```python
from build123d import *

# Parameters (mm, degrees)
BOSS_EXTRUDE1_DEPTH = 30
CUT_EXTRUDE1_DEPTH  = 59
SKETCH4_W           = 36.590571665
SKETCH4_H           = 16.65
BOSS_EXTRUDE2_DEPTH = 9
SKETCH5_W           = 22.6
SKETCH5_H           = 11.85
CUT_EXTRUDE2_DEPTH  = 4.3
CUT_EXTRUDE3_DEPTH  = 10.2
BOSS_EXTRUDE3_DEPTH = 27
SKETCH9_R           = 1.5875
BOSS_EXTRUDE5_DEPTH = 2.54
SKETCH11_R          = 1.7526
CUT_EXTRUDE4_DEPTH  = 16
FILLET1_R           = 2


with BuildPart() as part:
    # Sketch1 → Boss-Extrude1 (new body)
    with BuildSketch(Plane.XY):
        Polygon((0, 50.21875), (0, 0), (82, 0), (82, 60), (44.352804008, 60), (37.500008496, 71.86939), (12.500002832, 71.86939), align=None)
    extrude(amount=BOSS_EXTRUDE1_DEPTH)

    # Sketch3 → Cut-Extrude1 (cut)
    with BuildSketch(Plane.XY.offset(30)):
        Polygon((42.909428335, 57.5), (36.056632823, 69.36939), (13.943378505, 69.36939), (2.5, 49.548877019), (2.5, 2.5), (79.5, 2.5), (79.5, 57.5), align=None)
    extrude(amount=-CUT_EXTRUDE1_DEPTH, mode=Mode.SUBTRACT)

    # Sketch4 → Boss-Extrude2 (add)
    with BuildSketch(Plane.XY.offset(30)):
        with Locations((61.204714168, 49.175)):
            Rectangle(SKETCH4_W, SKETCH4_H)
    extrude(amount=-BOSS_EXTRUDE2_DEPTH)

    # Sketch5 → Cut-Extrude2 (cut)
    with BuildSketch(Plane(origin=(0, 0, 21), x_dir=(-1, 0, 0), z_dir=(0, 0, -1))):
        with Locations((-60.82763, 51.575)):
            Rectangle(SKETCH5_W, SKETCH5_H)
    extrude(amount=-CUT_EXTRUDE2_DEPTH, mode=Mode.SUBTRACT)

    # Sketch6 → Cut-Extrude3 (cut)
    with BuildSketch(Plane(origin=(0, 0, 25.3), x_dir=(-1, 0, 0), z_dir=(0, 0, -1))):
        with BuildLine():
            Line((-61.72763, 54.15), (-60.723855071, 54.15))
            ThreePointArc((-60.723855071, 54.15), (-49.52763, 51.55), (-60.723855071, 48.95))
            Line((-60.723855071, 48.95), (-61.72763, 48.95))
            ThreePointArc((-61.72763, 48.95), (-64.32763, 51.55), (-61.72763, 54.15))
        make_face()
    extrude(amount=-CUT_EXTRUDE3_DEPTH, mode=Mode.SUBTRACT)

    # Sketch8 → Boss-Extrude3 (add)
    with BuildSketch(Plane.XY.offset(30)):
        Polygon((13.943378505, 69.36939), (2.5, 49.548877019), (2.5, 2.5), (79.5, 2.5), (79.5, 40.85), (77.5, 40.85), (77.5, 4.5), (4.5, 4.5), (4.5, 49.012978634), (15.098079043, 67.36939), (34.901932285, 67.36939), (40.909428335, 56.964101615), (40.909428335, 55.471773493), (42.909428335, 55.471773493), (42.909428335, 57.5), (36.056632823, 69.36939), align=None)
    extrude(amount=-BOSS_EXTRUDE3_DEPTH)

    # Sketch9 → Boss-Extrude5 (add)
    # profile 1 of 3: a face of its own
    with BuildSketch(Plane.XY.offset(30)):
        with BuildLine():
            Line((4.5, 49.012978634), (4.5, 45.39891))
            Line((4.5, 45.39891), (8.89, 45.39891))
            ThreePointArc((8.89, 45.39891), (12.1205, 48.62941), (8.89, 51.85991))
            Line((8.89, 51.85991), (6.14367659, 51.85991))
            Line((6.14367659, 51.85991), (4.5, 49.012978634))
        make_face()
        with Locations((8.89, 48.62941)):
            Circle(SKETCH9_R, mode=Mode.SUBTRACT)
    # profile 2 of 3: a face of its own
    with BuildSketch(Plane.XY.offset(30)):
        with BuildLine():
            Line((4.5, 4.5), (12.1205, 4.5))
            Line((12.1205, 4.5), (12.1205, 8.89))
            ThreePointArc((12.1205, 8.89), (11.174308457, 11.174308457), (8.89, 12.1205))
            Line((8.89, 12.1205), (4.5, 12.1205))
            Line((4.5, 12.1205), (4.5, 4.5))
        make_face()
        with Locations((8.89, 8.89)):
            Circle(SKETCH9_R, mode=Mode.SUBTRACT)
    # profile 3 of 3: a face of its own
    with BuildSketch(Plane.XY.offset(30)):
        with BuildLine():
            Line((77.5, 4.5), (77.5, 40.85))
            Line((77.5, 40.85), (68.00821278, 40.85))
            Line((68.00821278, 40.85), (42.909428335, 40.85))
            Line((42.909428335, 40.85), (42.909428335, 30.90234))
            Line((42.909428335, 30.90234), (68.00821278, 30.90234))
            Line((68.00821278, 30.90234), (68.00821278, 14.90234))
            Line((68.00821278, 14.90234), (44.3405, 14.90234))
            Line((44.3405, 14.90234), (41.11, 14.90234))
            ThreePointArc((41.11, 14.90234), (36.858633615, 13.141366385), (35.09766, 8.89))
            Line((35.09766, 8.89), (35.09766, 4.5))
            Line((35.09766, 4.5), (44.3405, 4.5))
            Line((44.3405, 4.5), (68.00821278, 4.5))
            Line((68.00821278, 4.5), (77.5, 4.5))
        make_face()
        with Locations((41.11, 8.89)):
            Circle(SKETCH9_R, mode=Mode.SUBTRACT)
    extrude(amount=-BOSS_EXTRUDE5_DEPTH)

    # Sketch11 → Cut-Extrude4 (cut)
    with BuildSketch(Plane(origin=(0, 0, 27.46), x_dir=(-1, 0, 0), z_dir=(0, 0, -1))):
        with Locations((-60.00821, 35)):
            Circle(SKETCH11_R)
        with Locations((-60.00821, 11)):
            Circle(SKETCH11_R)
    extrude(amount=-CUT_EXTRUDE4_DEPTH, mode=Mode.SUBTRACT)

    # Fillet1
    fillet1_edges = [part.edges().sort_by_distance(p)[0] for p in [
        (60.723855071, 48.95, 27.65),
        (60.723855071, 54.15, 27.65),
    ]]
    fillet(fillet1_edges, radius=FILLET1_R)


solid = part.part
```
Geometry check sheet. Reference: the model listing, model coordinates, mm. A direction names the side the tool comes from. Coordinates: 2 decimals unless noted, no trailing zeros. Loops run counter-clockwise (first coordinate to the right, second up) from the corner with the lowest first, then second, coordinate; pieces in that order, holes last. Notation, with made-up numbers: (2, 24.25) -> (51, 24.25) arc R20 ccw to (51, 55.25) -> close; hole circle Ø1 at (1.5, 18.25). An arc over 180 degrees is marked (long way). Put each result on its own line as item: value.
1) Cross-section at C-C on z = 24. Record the boundary of the cut face in (x, y).
Result set:
outline: (0, 0) -> (82, 0) -> (82, 60) -> (44.35, 60) -> (37.5, 71.87) -> (12.5, 71.87) -> (0, 50.22) -> close; hole (4.5, 4.5) -> (77.5, 4.5) -> (77.5, 40.85) -> (42.91, 40.85) -> (42.91, 55.47) -> (40.91, 55.47) -> (40.91, 56.96) -> (34.9, 67.37) -> (15.1, 67.37) -> (4.5, 49.01) -> close; hole (49.53, 45.65) -> (72.13, 45.65) -> (72.13, 57.5) -> (49.53, 57.5) -> close
2) Thickness scan on line 1 (Y direction, x = 69, z = 24); line 2 (X direction, y = 8.5, z = 10); line 3 (X direction, y = 48, z = 20). Record the ranges inside material, lowest first.
Result set:
line 1: y = 0 to 4.5, 40.85 to 45.65, 57.5 to 60
line 2: x = 0 to 4.5, 77.5 to 82
line 3: x = 0 to 4.5, 79.5 to 82
3) Cross-section at D-D on x = 26. Record the boundary of the cut face in (y, z).
Result set:
outline: (0, 0) -> (2.5, 0) -> (2.5, 3) -> (4.5, 3) -> (4.5, 30) -> (0, 30) -> close; (67.37, 3) -> (69.37, 3) -> (69.37, 0) -> (71.87, 0) -> (71.87, 30) -> (67.37, 30) -> close
4) Gauge pin test, flat ends, axial feed: pin 1 Ø0.7 at (y, z) = (56, 15) entering from -X; pin 2 Ø4 at (x, z) = (62, 20) entering from +Y; pin 3 Ø8.5 at (x, y) = (10, 9) entering from -Z. Record the tip position at first contact, or that the pin passes through.
Result set:
pin 1: stops at x = 3.14
pin 2: stops at y = 60
pin 3: stops at z = 27.46
5) Release check for a two-part mould opening along Y. For faces 1 (the flat face through (0, 25, 15)), 2 (the cylindrical face through (9.62, 7.48, 28.75)), 3 (the flat face through (25, 71.869, 15)) record: released by +Y, released by -Y, zero draft, split by the parting line, or undercut.
Result set:
face 1: zero draft
face 2: undercut
face 3: released by +Y
6) Tool access check on faces 4 (the flat face through (42, 55.472, 17)), 5 (the flat face through (40, 0, 15)), 6 (the flat face through (35, 4, 3)). Record the directions out of +Z, -Z, +X, -X, +Y, -Y that give a thin tool (end or side, any length) a straight path to the whole face; none if there is none.
Result set:
face 4: +Z, -Z
face 5: +Z, -Z, +X, -X, -Y
face 6: -Z
7) Cross-section at B-B on x = 67. Record the boundary of the cut face in (y, z).
Result set:
outline: (0, 0) -> (2.5, 0) -> (2.5, 3) -> (4.5, 3) -> (4.5, 27.46) -> (14.9, 27.46) -> (14.9, 30) -> (0, 30) -> close; (30.9, 27.46) -> (40.85, 27.46) -> (40.85, 21) -> (45.65, 21) -> (45.65, 25.3) -> (57.5, 25.3) -> (57.5, 0) -> (60, 0) -> (60, 30) -> (30.9, 30) -> close
8) Cross-section at A-A on z = 9.5. Record the boundary of the cut face in (x, y), plus the area to 3 significant figures.
Result set:
outline: (0, 0) -> (82, 0) -> (82, 60) -> (44.35, 60) -> (37.5, 71.87) -> (12.5, 71.87) -> (0, 50.22) -> close; hole (4.5, 4.5) -> (77.5, 4.5) -> (77.5, 40.85) -> (79.5, 40.85) -> (79.5, 57.5) -> (42.91, 57.5) -> (42.91, 55.47) -> (40.91, 55.47) -> (40.91, 56.96) -> (34.9, 67.37) -> (15.1, 67.37) -> (4.5, 49.01) -> close
area: 1,140 mm^2
